Can you work these out from the model? Positions are in its coordinate system, mm. Face numbers are marked on the shaded views. A direction names the side the tool comes from. Coordinates: 2 decimals unless noted, no trailing zeros. Write each loop counter-clockwise with the first axis right and the second up, starting at its lowest first coordinate (ties: lowest second). Pieces come first, ordered by that corner, then holes.
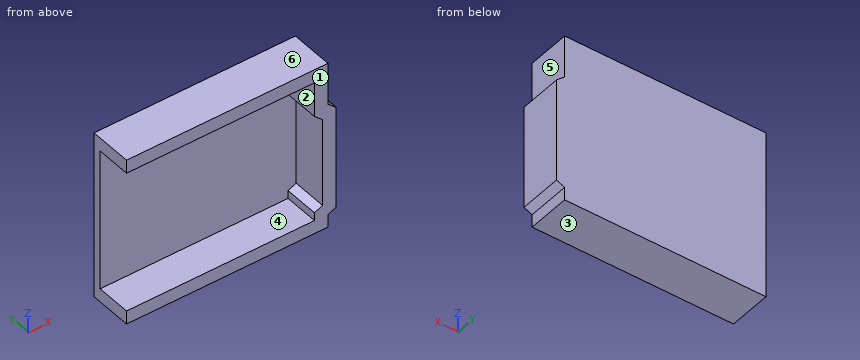
```python
from build123d import *

# Parameters (mm, degrees)
F1_DEPTH = 16
F0_W     = 5
F0_H     = 53
F2_DEPTH = 1.7
F3_DEPTH = 3
F4_DEPTH = 3


with BuildPart() as f1:
    # F0 (on Front) → F1 (new body)
    with BuildSketch(Plane.XZ):
        Polygon((-5, 0), (0, 0), (65, 0), (65, -13), (68, -15.645751), (68, -48.645751), (65, -50), (65, -53), (0, -53), (-5, -53), (-5, -58), (70, -58), (70, -53.228757), (73, -51.874508), (73, -13.38867), (70, -10.742919), (70, 5), (-5, 5), align=None)
    extrude(amount=F1_DEPTH)

    # F0 (on Front) → F2 (join)
    with BuildSketch(Plane.XZ):
        Polygon((-5, 0), (0, 0), (65, 0), (65, -13), (68, -15.645751), (68, -48.645751), (65, -50), (65, -53), (0, -53), (-5, -53), (-5, -58), (70, -58), (70, -53.228757), (73, -51.874508), (73, -13.38867), (70, -10.742919), (70, 5), (-5, 5), align=None)
        with Locations((-2.5, -26.5)):
            Rectangle(F0_W, F0_H)
    extrude(amount=F2_DEPTH)

    # F0 (on Front) → F3 (join)
    with BuildSketch(Plane.XZ):
        Polygon((-5, 0), (0, 0), (65, 0), (65, -13), (68, -15.645751), (68, -48.645751), (65, -50), (65, -53), (0, -53), (-5, -53), (-5, -58), (70, -58), (70, -53.228757), (73, -51.874508), (73, -13.38867), (70, -10.742919), (70, 5), (-5, 5), align=None)
        with Locations((-2.5, -26.5)):
            Rectangle(F0_W, F0_H)
    extrude(amount=F3_DEPTH)

    # F0 (on Front) → F4 (join)
    with BuildSketch(Plane.XZ):
        Polygon((65, 0), (0, 0), (0, -53), (65, -53), (65, -50), (68, -48.645751), (68, -15.645751), (65, -13), align=None)
    extrude(amount=F4_DEPTH)


solid = f1.part
```
1. If we section it at B-B, the plane x = 57: List the corners of the cut face in (y, z) for me, plus the area to 3 significant figures.
2. I'm going to push flat-ended pins straight in: P1, Ø4, axis at x = 17, z = -36.5, coming from the -Y side; P2, Ø5, axis at y = -11.5, z = -6.5, coming from the +X side; P3, Ø2.5, axis at y = -12.5, z = -51, coming from the -X side. Where does each tip first touch, or does it pass through?
3. If I drill on L1, parallel to Z at x = 5, y = -9.25; L2, parallel to X at y = -6, z = -10; L3, parallel to Y at x = 57, z = -49, over which ranges is the centre line in solid material (lowest first)?
4. We'd pull the mould along Z, two halves only. Please class the marked faces 1, 2 and 3: released by +Z, released by -Z, zero draft, split by the parting line, or undercut.
5. If we section it at A-A, the plane y = -7.5: List the corners of the cut face in (x, z) for me, plus the area to 3 significant figures.
6. If we section it at C-C, the plane z = -41.5: List the corners of the cut face in (x, y) for me, plus the area to 3 significant figures.
7. Which directions (+Z, -Z, +X, -X, +Y, -Y) give clear straight access to the entire face, cutting with the end or side of a thin tool? Please do the marked faces 4, 5 and 6.
8. If we section it at D-D, the plane z = -6: List the corners of the cut face in (x, y) for me, plus the area to 3 significant figures.
Answers:
1. outline: (-16, -58) - (0, -58) - (0, 5) - (-16, 5) - (-16, 0) - (-3, 0) - (-3, -53) - (-16, -53) - close
1. area: 319 mm2
2. P1: stops at y = -3
2. P2: stops at x = 70
2. P3: stops at x = 65
3. L1: z = -58 to -53, 0 to 5
3. L2: x = 65 to 70
3. L3: y = -3 to 0
4. face 1: zero draft
4. face 2: undercut
4. face 3: released by -Z
5. outline: (-5, -58) - (70, -58) - (70, -53.23) - (73, -51.87) - (73, -13.39) - (70, -10.74) - (70, 5) - (-5, 5) - (-5, 0) - (65, 0) - (65, -13) - (68, -15.65) - (68, -48.65) - (65, -50) - (65, -53) - (-5, -53) - close
5. area: 1,030 mm2
6. outline: (-5, -3) - (68, -3) - (68, -16) - (73, -16) - (73, 0) - (-5, 0) - close
6. area: 299 mm2
7. face 4: -X, -Y
7. face 5: +Z, +X, +Y, -Y
7. face 6: +Z, +X, -X, +Y, -Y
8. outline: (-5, -3) - (65, -3) - (65, -16) - (70, -16) - (70, 0) - (-5, 0) - close
8. area: 290 mm2
